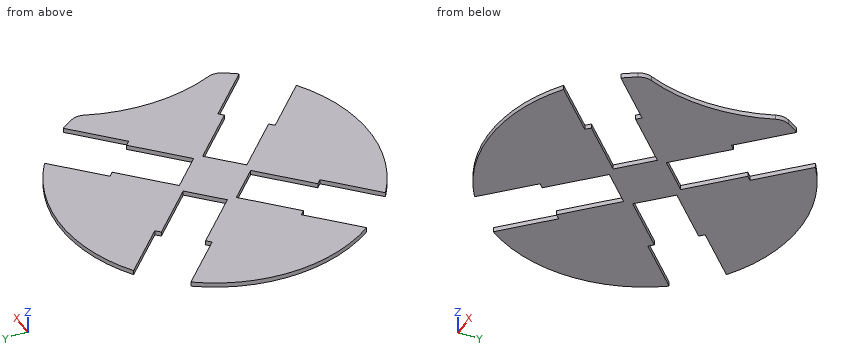
```python
from build123d import *

# Parameters (mm, degrees)
CROQUIS1_R              = 100
SALIENTE_EXTRUIR1_DEPTH = 3
CROQUIS3_R              = 110
CORTAR_EXTRUIR1_DEPTH   = 3
REDONDEO1_R             = 10
CORTAR_EXTRUIR2_DEPTH   = 142.453172607


with BuildPart() as part:
    # Croquis1 → Saliente-Extruir1 (new body)
    with BuildSketch(Plane.XY):
        Circle(CROQUIS1_R)
    extrude(amount=SALIENTE_EXTRUIR1_DEPTH)

    # Croquis3 → Cortar-Extruir1 (cut)
    with BuildSketch(Plane.XY.offset(3)):
        with Locations((190, 0)):
            Circle(CROQUIS3_R)
    extrude(amount=-CORTAR_EXTRUIR1_DEPTH, mode=Mode.SUBTRACT)

    # Redondeo1
    redondeo1_edges = [part.edges().sort_by_distance(p)[0] for p in [
        (89.473684211, -44.659375654, 1.5),
        (89.473684211, 44.659375654, 1.5),
    ]]
    fillet(redondeo1_edges, radius=REDONDEO1_R)

    # Croquis4 → Cortar-Extruir2 (cut, through all)
    with BuildSketch(Plane.XY.offset(3)):
        Polygon((-58.513086143, -82.908270094), (-83.261823485, -58.159532753), (-53.916892065, -28.814601333), (-51.088464941, -31.643028458), (-22.097086912, -2.651650429), (-3.00520382, -21.743533521), (-31.996581849, -50.73491155), (-29.168154724, -53.563338675), align=None)
        Polygon((-82.908270094, 58.513086143), (-53.563338675, 29.168154724), (-50.73491155, 31.996581849), (-21.743533521, 3.00520382), (-2.651650429, 22.097086912), (-31.643028458, 51.088464941), (-28.814601333, 53.916892065), (-58.159532753, 83.261823485), align=None)
        Polygon((58.513086143, 82.908270094), (29.168154724, 53.563338675), (31.996581849, 50.73491155), (3.00520382, 21.743533521), (22.097086912, 2.651650429), (51.088464941, 31.643028458), (53.916892065, 28.814601333), (83.261823485, 58.159532753), align=None)
        Polygon((82.908270094, -58.513086143), (53.563338675, -29.168154724), (50.73491155, -31.996581849), (21.743533521, -3.00520382), (2.651650429, -22.097086912), (31.643028458, -51.088464941), (28.814601333, -53.916892065), (58.159532753, -83.261823485), align=None)
    extrude(amount=-CORTAR_EXTRUIR2_DEPTH, mode=Mode.SUBTRACT)


solid = part.part
```
Model file for the job. Use its own axes, mm. Round coordinates to 2 decimals unless told otherwise and drop trailing zeros. Order: outer loops, then holes, each group sorted by start corner. A loop starts at its lowest first (then second) coordinate and runs counter-clockwise, first axis right, second up. Notation, with made-up numbers: M -25,72.25 L -9,72.25 A21 cw -9,86.25 Z; hole C 64.25,52 d4. An arc over 180 degrees is marked long. Use CSV: the item, a comma, the result in double quotes.
Item 1: Saw through at A-A (y = -18.5). List the corners of the cut face in (x, z), plus the area to 3 significant figures.
Worked answers:
outline,"M -98.27,0 L -37.95,0 L -37.95,3 L -98.27,3 Z; M -6.25,0 L 6.25,0 L 6.25,3 L -6.25,3 Z; M 37.24,0 L 81.57,0 L 81.57,3 L 37.24,3 Z"
area,"351 mm²"
Item 2: Saw through at C-C (y = 64.5). List the corners of the cut face in (x, z).
Worked answers:
outline,"M -39.4,0 L 40.1,0 L 40.1,3 L -39.4,3 Z"
Item 3: Saw through at B-B (x = -46.5). List the corners of the cut face in (y, z).
Worked answers:
outline,"M -88.53,0 L -70.9,0 L -70.9,3 L -88.53,3 Z; M -27.05,0 L 27.76,0 L 27.76,3 L -27.05,3 Z; M 71.6,0 L 88.53,0 L 88.53,3 L 71.6,3 Z"
Item 4: Saw through at D-D (y = -70). List the corners of the cut face in (x, z), plus the area to 3 significant figures.
Worked answers:
outline,"M -45.6,0 L 44.9,0 L 44.9,3 L -45.6,3 Z"
area,"272 mm²"
Item 5: Probe probe 1 along X at (y, z) = (-51.5, 1); probe 2 along X at (y, z) = (20, 2.2); probe 3 along Y at (x, z) = (-56, 1.75). List the from-to ranges inside material, lowest first.
Worked answers:
probe 1,"-85.72 to -76.6, -31.23 to 31.23, 75.9 to 85.72"
probe 2,"-97.98 to -38.74, -4.75 to 4.75, 39.45 to 81.83"
probe 3,"-82.85 to -80.4, -30.9 to 31.6, 81.1 to 82.85"
